from build123d import *

# Parameters (mm, degrees)
BOSS_EXTRUDE1_DEPTH = 5
SKETCH3_W           = 5
SKETCH3_H           = 70
BOSS_EXTRUDE3_DEPTH = 20.7
SKETCH2_W           = 12.8
SKETCH2_H           = 13.045671514
BOSS_EXTRUDE4_DEPTH = 3
SKETCH4_R           = 4.5
BOSS_EXTRUDE5_DEPTH = 5


with BuildPart() as part:
    # Sketch1 → Boss-Extrude1 (new body)
    with BuildSketch(Plane.XY):
        with BuildLine():
            Line((-90, -50), (90, -50))
            ThreePointArc((90, -50), (100.606601718, -45.606601718), (105, -35))
            Line((105, -35), (105, 35))
            ThreePointArc((105, 35), (100.606601718, 45.606601718), (90, 50))
            Line((90, 50), (-90, 50))
            ThreePointArc((-90, 50), (-100.606601718, 45.606601718), (-105, 35))
            Line((-105, 35), (-105, -35))
            ThreePointArc((-105, -35), (-100.606601718, -45.606601718), (-90, -50))
        make_face()
    extrude(amount=BOSS_EXTRUDE1_DEPTH)

    # Sketch3 → Boss-Extrude3 (add)
    with BuildSketch(Plane.XY.offset(5)):
        with Locations((102.5, 0)):
            Rectangle(SKETCH3_W, SKETCH3_H)
        with Locations((-102.5, 0)):
            Rectangle(SKETCH3_W, SKETCH3_H)
    extrude(amount=BOSS_EXTRUDE3_DEPTH)

    # Sketch2 → Boss-Extrude4 (add)
    with BuildSketch(Plane.XY.offset(5)):
        with Locations((-67.473686504, 43.477164243)):
            Rectangle(SKETCH2_W, SKETCH2_H)
        with Locations((-4.473686504, 43.477164243)):
            Rectangle(SKETCH2_W, SKETCH2_H)
        with Locations((58.526313496, 43.477164243)):
            Rectangle(SKETCH2_W, SKETCH2_H)
        with Locations((-67.473686504, -43.477164243)):
            Rectangle(SKETCH2_W, SKETCH2_H)
        with Locations((-4.473686504, -43.477164243)):
            Rectangle(SKETCH2_W, SKETCH2_H)
        with Locations((58.526313496, -43.477164243)):
            Rectangle(SKETCH2_W, SKETCH2_H)
    extrude(amount=BOSS_EXTRUDE4_DEPTH)

    # Sketch4 → Boss-Extrude5 (add)
    with BuildSketch(Plane.XY.offset(8)):
        with Locations(Location((-67.473686504, 43.477164243, 0), (0, 0, 180))):
            Circle(SKETCH4_R)
        with Locations((-4.473686504, 43.477164243)):
            Circle(SKETCH4_R)
        with Locations((58.526313496, 43.477164243)):
            Circle(SKETCH4_R)
        with Locations(Location((58.526313496, -43.477164243, 0), (0, 0, 180))):
            Circle(SKETCH4_R)
        with Locations(Location((-4.473686504, -43.477164243, 0), (0, 0, 180))):
            Circle(SKETCH4_R)
        with Locations(Location((-67.473686504, -43.477164243, 0), (0, 0, 180))):
            Circle(SKETCH4_R)
    extrude(amount=BOSS_EXTRUDE5_DEPTH)


solid = part.part
Here's how the part is built. I have some questions about the finished solid (model axes, mm). A direction names the side the tool comes from. Give positions to 0.01 mm unless a question says otherwise; leave off trailing zeros. Order: outer loops, then holes, each group sorted by start corner. A loop starts at its lowest first (then second) coordinate and runs counter-clockwise, first axis right, second up. Notation, with made-up numbers: (50, -36.75) -> (73, -36.75) arc R21 cw to (73, -32.75) -> close; hole circle Ø8 at (-23.75, 52). An arc over 180 degrees is marked (long way). One line per item, written item: value. Start each with the question number.
1. Imagine slicing it at B-B, the plane y = -28.5. List the corners of the cut face in (x, z) for me.
2. Imagine slicing it at D-D, the plane x = 10. List the corners of the cut face in (y, z) for me.
3. Imagine slicing it at A-A, the plane z = 23.5. List the corners of the cut face in (x, y) for me.
4. I need wall thicknesses on probe 1 along X at (y, z) = (-39.5, 6.5); probe 2 along X at (y, z) = (-34, 7.25); probe 3 along Z at (x, y) = (-74, -28). Which ranges of each line are inside material? Lowest first, please. Write a range as from..to.
5. For faces 1 (the face through (-103, 35, 15)), 2 (the face through (100, 0, 15)), 3 (the face through (-103, -35, 15)), 4 (the face through (-72, 45, 8)), which set-ups out of +Z, -Z, +X, -X, +Y, -Y let a thin tool reach every point of the face, with its end or its side?
6. We'd pull the mould along Y, two halves only. Please class faces 5 (the face through (-5, 44, 13)), 6 (the face through (1, 50, 3)), 7 (the face through (-63.9, -40.74, 10.46)): released by +Y, released by -Y, zero draft, split by the parting line, or undercut.
7. Will these pins go through, and if not, where does the flat tip stop? pin 1 Ø3.5 at (y, z) = (-45.5, 7) entering from +X; pin 2 Ø1 at (x, y) = (78.5, -15.5) entering from +Z; pin 3 Ø4 at (x, z) = (103, 20) entering from +Y.
8. Imagine slicing it at C-C, the plane x = 60. List the corners of the cut face in (y, z) for me, plus the area to 3 significant figures.
Values follow:
1. outline: (-105, 0) -> (105, 0) -> (105, 25.7) -> (100, 25.7) -> (100, 5) -> (-100, 5) -> (-100, 25.7) -> (-105, 25.7) -> close
2. outline: (-50, 0) -> (50, 0) -> (50, 5) -> (-50, 5) -> close
3. outline: (-105, -35) -> (-100, -35) -> (-100, 35) -> (-105, 35) -> close; (100, -35) -> (105, -35) -> (105, 35) -> (100, 35) -> close
4. probe 1: x = -73.87..-61.07, -10.87..1.93, 52.13..64.93
4. probe 2: x = -105..-100, 100..105
4. probe 3: z = 0..5
5. face 1: +Z, +X, -X, +Y
5. face 2: +Z, +Y, -Y
5. face 3: +Z, +X, -X, -Y
5. face 4: +Z
6. face 5: zero draft
6. face 6: released by +Y
6. face 7: undercut
7. pin 1: stops at x = 64.93
7. pin 2: stops at z = 5
7. pin 3: stops at y = 35
8. outline: (-50, 0) -> (50, 0) -> (50, 8) -> (47.73, 8) -> (47.73, 13) -> (39.23, 13) -> (39.23, 8) -> (36.95, 8) -> (36.95, 5) -> (-36.95, 5) -> (-36.95, 8) -> (-39.23, 8) -> (-39.23, 13) -> (-47.73, 13) -> (-47.73, 8) -> (-50, 8) -> close
8. area: 663 mm2
